```python
from build123d import *

# Parameters (mm, degrees)
SKETCH_1_W      = 40
SKETCH_1_H      = 12.5
SKETCH_1_R      = 2.025
EXTRUDE_1_DEPTH = 1.5
FILLET_1_R      = 2


with BuildPart() as part:
    # 草图1 → 凸台-拉伸1 (new body, symmetric)
    with BuildSketch(Plane.XY):
        Rectangle(SKETCH_1_W, SKETCH_1_H)
        with Locations((-12.5, 0)):
            Circle(SKETCH_1_R, mode=Mode.SUBTRACT)
        with Locations((12.5, 0)):
            Circle(SKETCH_1_R, mode=Mode.SUBTRACT)
    extrude(amount=EXTRUDE_1_DEPTH, both=True)

    # 圆角1
    fillet_1_edges = [part.edges().sort_by_distance(p)[0] for p in [
        (20, -6.25, 0),
        (-20, -6.25, 0),
        (-20, 6.25, 0),
        (20, 6.25, 0),
    ]]
    fillet(fillet_1_edges, radius=FILLET_1_R)


solid = part.part
```
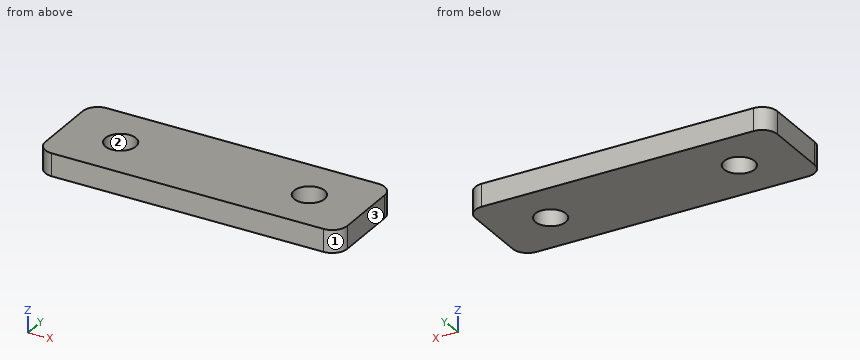
Model file for the job. Use its own axes, mm. Face numbers are marked on the shaded views. Coordinates: 2 decimals unless noted, no trailing zeros. Loops run counter-clockwise (first coordinate to the right, second up) from the corner with the lowest first, then second, coordinate; pieces in that order, holes last. Notation, with made-up numbers: (25, -18) - (30, -18) arc R22 ccw to (30, -12) - close; hole circle Ø11 at (7, -26). An arc over 180 degrees is marked (long way). Write item = value, one per line. Start each with the question number.
Item 1: Saw through at A-A, the plane x = 12.5. List the corners of the cut face in (y, z) (3 decimals).
Item 2: Saw through at D-D, the plane y = 1.5. List the corners of the cut face in (x, z), then the cut area to 3 significant figures.
Item 3: Drop a flat-ended pin along its axis: pin 1 Ø2.5 at (x, y) = (-12.5, 0) entering from +Z. Give the stop position or say it passes through.
Item 4: Pull direction Y, two halves, no side cores. Call the marked faces 1, 2 and 3: +Y half, -Y half, draft (parallel to the pull), parting line (faces both ways), or undercut.
Item 5: Saw through at C-C, the plane z = -1.05. List the corners of the cut face in (x, y) (3 decimals).
Item 6: Wall check: probe 1 along Y at (x, z) = (12.5, -0.3) (3 decimals); probe 2 along X at (y, z) = (1, 0.1); probe 3 along X at (y, z) = (0.25, -1.05). Give the ranges that are in metal, low to high. Write a range as [from, to].
Item 7: Saw through at B-B, the plane y = 0. List the corners of the cut face in (x, z) (3 decimals).
Answers:
q1.outline = (-6.25, -1.5) - (-2.025, -1.5) - (-2.025, 1.5) - (-6.25, 1.5) - close; (2.025, -1.5) - (6.25, -1.5) - (6.25, 1.5) - (2.025, 1.5) - close
q2.outline = (-20, -1.5) - (-13.86, -1.5) - (-13.86, 1.5) - (-20, 1.5) - close; (-11.14, -1.5) - (11.14, -1.5) - (11.14, 1.5) - (-11.14, 1.5) - close; (13.86, -1.5) - (20, -1.5) - (20, 1.5) - (13.86, 1.5) - close
q2.area = 104 mm2
q3.pin_1 = through
q4.face_1 = -Y half
q4.face_2 = undercut
q4.face_3 = draft
q5.outline = (-20, -4.25) arc R2 ccw to (-18, -6.25) - (18, -6.25) arc R2 ccw to (20, -4.25) - (20, 4.25) arc R2 ccw to (18, 6.25) - (-18, 6.25) arc R2 ccw to (-20, 4.25) - close; hole circle Ø4.05 at (-12.5, 0); hole circle Ø4.05 at (12.5, 0)
q6.probe_1 = [-6.25, -2.025], [2.025, 6.25]
q6.probe_2 = [-20, -14.26], [-10.74, 10.74], [14.26, 20]
q6.probe_3 = [-20, -14.51], [-10.49, 10.49], [14.51, 20]
q7.outline = (-20, -1.5) - (-14.525, -1.5) - (-14.525, 1.5) - (-20, 1.5) - close; (-10.475, -1.5) - (10.475, -1.5) - (10.475, 1.5) - (-10.475, 1.5) - close; (14.525, -1.5) - (20, -1.5) - (20, 1.5) - (14.525, 1.5) - close
